Here's the drawing with two shaded views (mm, measured from the low corner). I have some questions. A direction names the side the tool comes from. Round coordinates to 2 decimals unless told otherwise and drop trailing zeros. Loops run counter-clockwise (first coordinate to the right, second up) from the corner with the lowest first, then second, coordinate; pieces in that order, holes last.
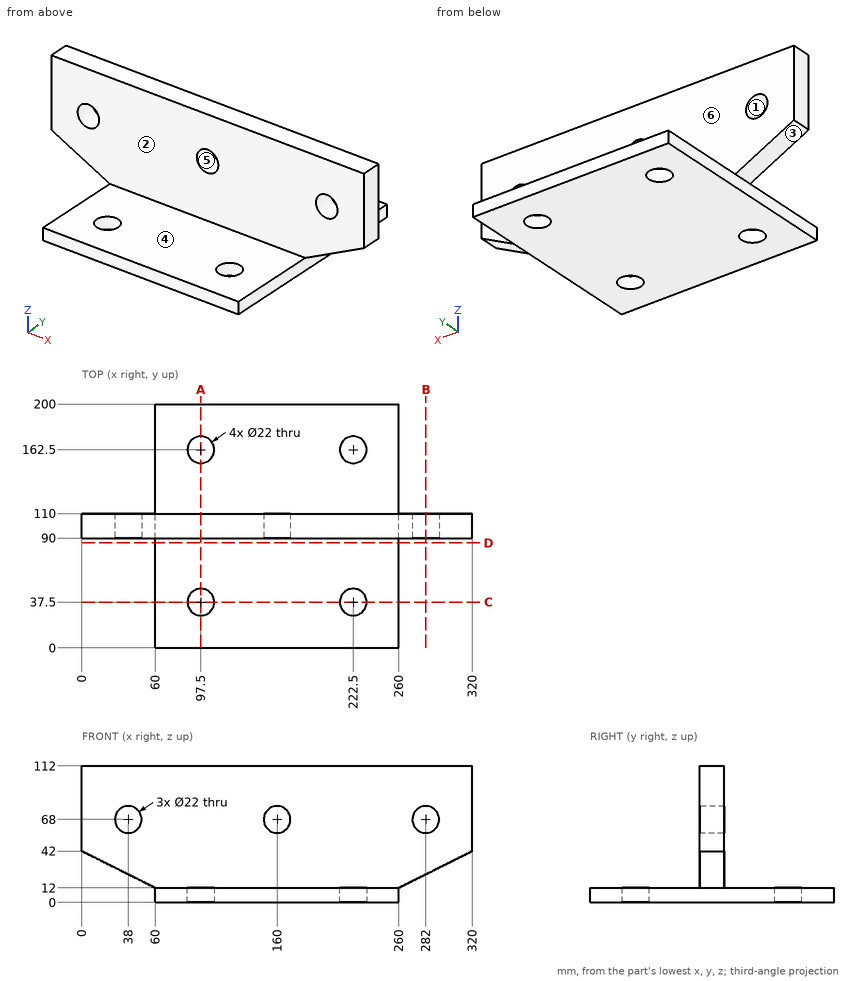
Item 1: If we section it at D-D, the plane y = 86: Please give me the cut outline in (x, z), then the cut area to 3 significant figures.
Results list:
outline: (60, 0) - (260, 0) - (260, 12) - (60, 12) - close
area: 2,400 mm2
Item 2: If I drill on line 1 along X through (y, z) = (98, 68); line 2 along X through (y, z) = (37, 8); line 3 along Y through (x, z) = (97.5, 4.5), over which ranges is the centre line in solid material (lowest first)?
Results list:
line 1: x = 0 to 27, 49 to 149, 171 to 271, 293 to 320
line 2: x = 60 to 86.51, 108.49 to 211.51, 233.49 to 260
line 3: y = 0 to 26.5, 48.5 to 151.5, 173.5 to 200
Item 3: If we section it at B-B, the plane x = 282: Please give me the cut outline in (y, z).
Results list:
outline: (90, 23) - (110, 23) - (110, 57) - (90, 57) - close; (90, 79) - (110, 79) - (110, 112) - (90, 112) - close
Item 4: If we section it at A-A, the plane x = 97.5: Please give me the cut outline in (y, z).
Results list:
outline: (0, 0) - (26.5, 0) - (26.5, 12) - (0, 12) - close; (48.5, 0) - (151.5, 0) - (151.5, 12) - (110, 12) - (110, 112) - (90, 112) - (90, 12) - (48.5, 12) - close; (173.5, 0) - (200, 0) - (200, 12) - (173.5, 12) - close
Item 5: Will these pins go through, and if not, where does the flat tip stop? pin 1 (3.5 mm diameter, centred on y = 146, z = 9, fed in from +X); pin 2 (6 mm diameter, centred on y = 50.5, z = 8, fed in from -X); pin 3 (12 mm diameter, centred on x = 100.5, y = 90, fed in from -Z); pin 4 (8 mm diameter, centred on x = 268, z = 53.5, fed in from -Y).
Results list:
pin 1: stops at x = 260
pin 2: stops at x = 60
pin 3: stops at z = 0
pin 4: stops at y = 90
Item 6: We'd pull the mould along X, two halves only. Please class the marked faces 1, 2 and 3: released by +X, released by -X, zero draft, split by the parting line, or undercut.
Results list:
face 1: undercut
face 2: zero draft
face 3: released by -X
Item 7: If we section it at C-C, the plane y = 37.5: Please give me the cut outline in (x, z), then the cut area to 3 significant figures.
Results list:
outline: (60, 0) - (86.5, 0) - (86.5, 12) - (60, 12) - close; (108.5, 0) - (211.5, 0) - (211.5, 12) - (108.5, 12) - close; (233.5, 0) - (260, 0) - (260, 12) - (233.5, 12) - close
area: 1,870 mm2
Item 8: For the marked faces 4, 5 and 6, which set-ups out of +Z, -Z, +X, -X, +Y, -Y let a thin tool reach every point of the face, with its end or its side?
Results list:
face 4: +Z, +X, -X, -Y
face 5: +Y, -Y
face 6: +Z, +X, -X, +Y
